Check sheet for the modelled part. Datum: model origin and axes. Units: mm. Face numbers are marked on the shaded views. A direction names the side the tool comes from. Give positions to 0.01 mm unless a question says otherwise; leave off trailing zeros. Write each loop counter-clockwise with the first axis right and the second up, starting at its lowest first coordinate (ties: lowest second). Pieces come first, ordered by that corner, then holes. Notation, with made-up numbers: M -1,-9 L 30,-9 A16 ccw 30,15 Z; hole C -5,48.5 d7. An arc over 180 degrees is marked long. Write item = value, one per line. Start each with the question number.
1) Scan lines: L1, parallel to Y at x = 5, z = -21.9; L2, parallel to Y at x = 6.75, z = -32.5; L3, parallel to Z at x = 5.75, y = -2.5. Record each from-to range of solid material in increasing order.
2) Gauge pin test, flat ends, axial feed: pin 1 (3 mm diameter, centred on x = 5.5, z = -27, fed in from -Y); pin 2 (3 mm diameter, centred on x = 5, z = 3.85, fed in from +Y); pin 3 (5 mm diameter, centred on x = 6.5, z = 4.5, fed in from +Y); pin 4 (1.5 mm diameter, centred on x = 2.5, y = -3, fed in from +Z). Record the tip position at first contact, or that the pin passes through.
3) Draft check along Y on the marked faces 1, 2, 3 and 4. Enter one of: pulls with the +Y half, pulls with the -Y half, needs draft (parallel to the pull), parting line crosses it, or undercut.
4) Set-up check for the marked faces 5 and 6: record each of +Z, -Z, +X, -X, +Y, -Y from which the full face is reachable in a straight line by a thin tool's end or side.
5) Sectioned sample at B-B, the plane y = -35. Record the cut outline in (x, z).
6) Sectioned sample at A-A, the plane x = 5. Record the cut outline in (y, z), then the cut area to 3 significant figures.
from build123d import *

# Parameters (mm, degrees)
BOSS_EXTRUDE1_DEPTH = 10
FILLET1_R           = 5
BOSS_EXTRUDE2_DEPTH = 4
SKETCH3_R           = 1.65
CUT_EXTRUDE1_DEPTH  = 55.081290223
BOSS_EXTRUDE3_DEPTH = 4
SKETCH5_R           = 1.65
CUT_EXTRUDE2_DEPTH  = 54.441556864
FILLET2_R           = 3
FILLET3_R           = 2


with BuildPart() as part:
    # Sketch1 → Boss-Extrude1 (new body)
    with BuildSketch(Plane(origin=(0, 0, 0), x_dir=(0, 0, -1), z_dir=(1, 0, 0))):
        Polygon((0, 0), (20, 0), (20, -30), (41.868360094, -30), (34.553508963, -9.90261169), (41.809544604, 31.248411326), (18.041278691, 31.248411326), align=None)
    extrude(amount=BOSS_EXTRUDE1_DEPTH)

    # Fillet1
    fillet1_edges = [part.edges().sort_by_distance(p)[0] for p in [
        (5, 31.248411326, -18.041278691),
        (5, 31.248411326, -41.809544604),
        (5, -9.90261169, -34.553508963),
        (5, -30, -41.868360094),
    ]]
    fillet(fillet1_edges, radius=FILLET1_R)

    # Sketch2 → Boss-Extrude2 (add)
    with BuildSketch(Plane.XZ):
        Polygon((0, -20), (0, 0), (0, 10), (10, 10), (10, 0), (10, -20), align=None)
    extrude(amount=-BOSS_EXTRUDE2_DEPTH)

    # Sketch3 → Cut-Extrude1 (cut, through all)
    with BuildSketch(Plane(origin=(0, 4, 0), x_dir=(1, 0, 0), z_dir=(0, 1, 0))):
        with Locations(Location((5, -3.845299462, 0), (0, 0, 270))):
            Circle(SKETCH3_R)
    extrude(amount=-CUT_EXTRUDE1_DEPTH, mode=Mode.SUBTRACT)

    # Sketch4 → Boss-Extrude3 (add)
    with BuildSketch(Plane.XY.offset(-20)):
        Polygon((0, 0), (0, -30), (0, -40), (10, -40), (10, -30), (10, 0), align=None)
    extrude(amount=-BOSS_EXTRUDE3_DEPTH)

    # Sketch5 → Cut-Extrude2 (cut, through all)
    with BuildSketch(Plane(origin=(0, 0, -24), x_dir=(-1, 0, 0), z_dir=(0, 0, -1))):
        with Locations((-5, -35)):
            Circle(SKETCH5_R)
    extrude(amount=-CUT_EXTRUDE2_DEPTH, mode=Mode.SUBTRACT)

    # Fillet2
    fillet2_edges = [part.edges().sort_by_distance(p)[0] for p in [
        (10, 2, 10),
        (0, 2, 10),
        (0, -40, -22),
        (10, -40, -22),
    ]]
    fillet(fillet2_edges, radius=FILLET2_R)

    # Fillet3
    fillet3_edges = [part.edges().sort_by_distance(p)[0] for p in [
        (0, -17.225730184, -37.218906116),
        (10, -17.225730184, -37.218906116),
        (0, 16.374205663, -9.453652047),
        (0, 31.248411326, -28.389403339),
        (0, 8.398475479, -37.780484407),
        (0, 30.578538345, -18.428030037),
        (0, 29.462349374, -39.680998857),
        (0, -27.867882182, -38.823380282),
        (10, 16.374205663, -9.453652047),
        (10, 8.398475479, -37.780484407),
        (10, 31.248411326, -28.389403339),
        (10, 30.578538345, -18.428030037),
        (10, 29.462349374, -39.680998857),
        (10, -27.867882182, -38.823380282),
        (0, -9.887239081, -34.729218682),
        (10, -9.887239081, -34.729218682),
        (0, -30, -29.36381003),
        (10, -30, -29.36381003),
    ]]
    fillet(fillet3_edges, radius=FILLET3_R)


solid = part.part
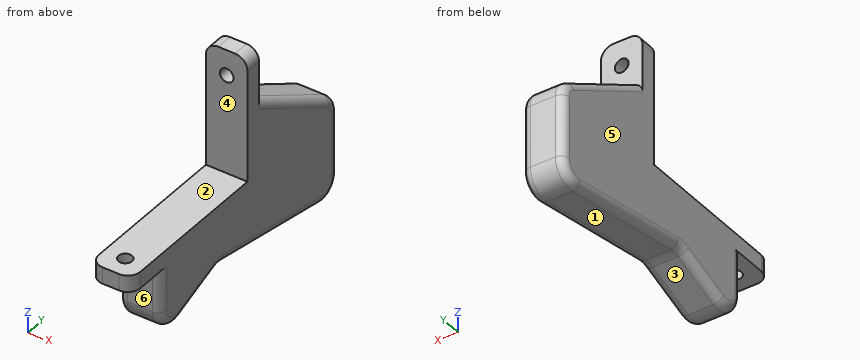
Data:
q1.L1 = -40 to -36.65, -33.35 to 31.25
q1.L2 = -30 to 31.25
q1.L3 = -35.86 to -20
q2.pin_1 = -30
q2.pin_2 = through
q2.pin_3 = 4
q2.pin_4 = -20
q3.face_1 = undercut
q3.face_2 = needs draft
q3.face_3 = undercut
q3.face_4 = pulls with the -Y half
q4.face_5 = +Z, -Z, -X, +Y, -Y
q4.face_6 = -Z, +X, -X, -Y
q5.outline = M 0,-24 L 3.35,-24 L 3.35,-20 L 0,-20 Z; M 6.65,-24 L 10,-24 L 10,-20 L 6.65,-20 Z
q6.outline = M -40,-24 L -36.65,-24 L -36.65,-20 L -40,-20 Z; M -33.35,-24 L -30,-24 L -30,-34.73 A5 ccw -23.29,-39.43 L -11.16,-35.01 A5 cw -8.58,-34.79 L 25.38,-40.77 A5 ccw 31.25,-35.85 L 31.25,-20.93 A5 ccw 28.75,-16.6 L 4,-2.31 L 4,2.2 L 0,2.2 L 0,-20 L -33.35,-20 Z; M 0,5.5 L 4,5.5 L 4,10 L 0,10 Z
q6.area = 1,490 mm2
